Design review of the part built by this model. Coordinates are the model's own, in mm. Face numbers are marked on the shaded views. Give positions to 0.01 mm unless a question says otherwise; leave off trailing zeros. Order: outer loops, then holes, each group sorted by start corner. A loop starts at its lowest first (then second) coordinate and runs counter-clockwise, first axis right, second up. Notation, with made-up numbers: M 64,31.5 L 116,31.5 A28 ccw 116,51.5 Z; hole C 56.5,1 d11. An arc over 180 degrees is marked long. Answer as a JSON object with one key per item and string values.
from build123d import *

# Parameters (mm, degrees)
SKETCH1_W           = 31.88
SKETCH1_H           = 7.82
BOSS_EXTRUDE1_DEPTH = 3.15
SHELL1_T            = -1.6
SKETCH2_R           = 1.475
SKETCH2_R_2         = 0.7
BOSS_EXTRUDE2_DEPTH = 1.35


with BuildPart() as part:
    # Sketch1 → Boss-Extrude1 (new body)
    with BuildSketch(Plane(origin=(0, 0, 0), x_dir=(1, 0, 0), z_dir=(0, 1, 0))):
        Rectangle(SKETCH1_W, SKETCH1_H)
    extrude(amount=-BOSS_EXTRUDE1_DEPTH)

    # Shell1
    shell1_openings = [part.faces().sort_by_distance(p)[0] for p in [
        (0, -3.15, 0),
    ]]
    offset(amount=SHELL1_T, openings=shell1_openings, kind=Kind.INTERSECTION)

    # Sketch2 → Boss-Extrude2 (add)
    # profile 1 of 3: a face of its own
    with BuildSketch(Plane.XZ.offset(1.6)):
        with Locations(Location((-7.97, 0, 0), (0, 0, 90))):
            Circle(SKETCH2_R)
        with Locations(Location((-7.97, 0, 0), (0, 0, 90))):
            Circle(SKETCH2_R_2, mode=Mode.SUBTRACT)
    # profile 2 of 3: a face of its own
    with BuildSketch(Plane.XZ.offset(1.6)):
        with Locations(Location((0, 0, 0), (0, 0, 90))):
            Circle(SKETCH2_R)
        with Locations(Location((0, 0, 0), (0, 0, 90))):
            Circle(SKETCH2_R_2, mode=Mode.SUBTRACT)
    # profile 3 of 3: a face of its own
    with BuildSketch(Plane.XZ.offset(1.6)):
        with Locations(Location((7.97, 0, 0), (0, 0, 90))):
            Circle(SKETCH2_R)
        with Locations(Location((7.97, 0, 0), (0, 0, 90))):
            Circle(SKETCH2_R_2, mode=Mode.SUBTRACT)
    extrude(amount=BOSS_EXTRUDE2_DEPTH)


solid = part.part
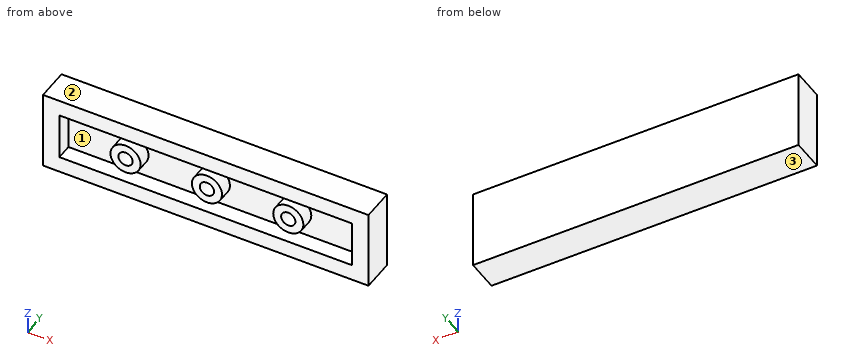
(1) Draft analysis for pull direction Z (two halves, no side actions). For the marked faces 1, 2 and 3, state which applies: +Z half, -Z half, draft (parallel to the pull), parting line (faces both ways), or undercut.
Checked values:
{"face 1": "undercut", "face 2": "+Z half", "face 3": "-Z half"}
(2) To check wall thickness, follow L1, parallel to Z at x = 7.97, y = -2.5 (3 decimals); L2, parallel to Z at x = 2.5, y = -2.4; L3, parallel to Z at x = -9, y = -1.7. State the ranges of each line that lie inside material, in increasing order. Write a range as from..to.
Checked values:
{"L1": "z = -3.91..-2.31, -1.475..-0.7, 0.7..1.475, 2.31..3.91", "L2": "z = -3.91..-2.31, 2.31..3.91", "L3": "z = -3.91..-2.31, -1.06..1.06, 2.31..3.91"}
(3) Insertion check: pin 1 (0.9 mm diameter, centred on x = -8.5, z = 0, fed in from -Y); pin 2 (1.1 mm diameter, centred on x = 0, z = 0, fed in from -Y). Each pin has a flat end and moves straight along its axis. Give the tip position at first contact, or say it passes through.
Checked values:
{"pin 1": "stops at y = -2.95", "pin 2": "stops at y = -1.6"}
(4) We need section B-B (x = -7.97). Write out the cut boundary in (y, z) (3 decimals).
Checked values:
{"outline": "M -3.15,-3.91 L 0,-3.91 L 0,3.91 L -3.15,3.91 L -3.15,2.31 L -1.6,2.31 L -1.6,1.475 L -2.95,1.475 L -2.95,0.7 L -1.6,0.7 L -1.6,-0.7 L -2.95,-0.7 L -2.95,-1.475 L -1.6,-1.475 L -1.6,-2.31 L -3.15,-2.31 Z"}
(5) We need section A-A (y = -2.65). Write out the cut boundary in (x, z) (3 decimals).
Checked values:
{"outline": "M -15.94,-3.91 L 15.94,-3.91 L 15.94,3.91 L -15.94,3.91 Z; C -7.97,0 d2.95; C 0,0 d2.95; C 7.97,0 d2.95; hole M -14.34,-2.31 L 14.34,-2.31 L 14.34,2.31 L -14.34,2.31 Z; hole C -7.97,0 d1.4; hole C 0,0 d1.4; hole C 7.97,0 d1.4"}
